The figure shows three views and two pictorial views of one solid part (mm, origin at its lowest corner). Answer the questions. A direction names the side the tool comes from. Round coordinates to 2 decimals unless told otherwise and drop trailing zeros. Write each loop counter-clockwise with the first axis right and the second up, starting at its lowest first coordinate (ties: lowest second). Pieces come first, ordered by that corner, then holes.
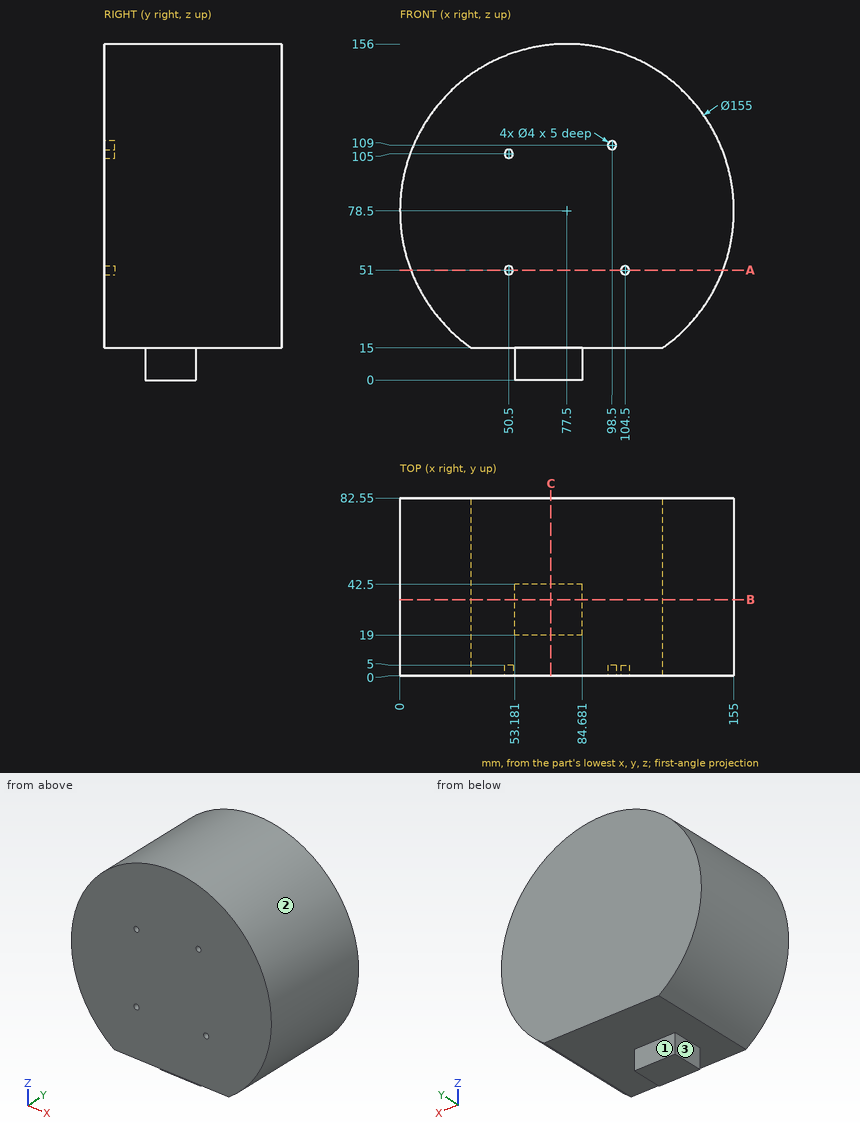
Q1. Section A-A (z = 51) is taken. Determine the outline of the cut face in (x, y).
Verdict:
outline: (5.04, 0) - (48.5, 0) - (48.5, 5) - (52.5, 5) - (52.5, 0) - (102.5, 0) - (102.5, 5) - (106.5, 5) - (106.5, 0) - (149.96, 0) - (149.96, 82.55) - (5.04, 82.55) - close
Q2. Section C-C (x = 70) is taken. Determine the outline of the cut face in (y, z).
Verdict:
outline: (0, 15) - (19, 15) - (19, 0) - (42.5, 0) - (42.5, 15) - (82.55, 15) - (82.55, 155.64) - (0, 155.64) - close
Q3. Section B-B (y = 35.5) is taken. Determine the outline of the cut face in (x, z).
Verdict:
outline: (33.07, 15) - (53.18, 15) - (53.18, 0) - (84.68, 0) - (84.68, 15) - (121.93, 15) arc R77.5 ccw (long way) to start
Q4. Straight lines are drawn through the part: probe 1 along Z at (x, y) = (50.5, 3.1) (1 decimal); probe 2 along Z at (x, y) = (77, 53); probe 3 along X at (y, z) = (2, 105). For each, find the intervals that lie inside material, in ascending order.
Verdict:
probe 1: z = 15 to 49, 53 to 103, 107 to 151.1
probe 2: z = 15 to 156
probe 3: x = 4.67 to 48.5, 52.5 to 150.33
Q5. Flat-ended cylindrical pins translate along their axes: pin 1 Ø2 at (x, y) = (125, 70.5) entering from -Z; pin 2 Ø4 at (x, z) = (82.5, 58.5) entering from -Y; pin 3 Ø4 at (y, z) = (41.5, 133) entering from -X; pin 4 Ø7.5 at (y, z) = (33.5, 8) entering from -X. Find the tip coordinate at first contact, or state that the pin passes through.
Verdict:
pin 1: stops at z = 16.5
pin 2: stops at y = 0
pin 3: stops at x = 20.49
pin 4: stops at x = 53.18
Q6. Which of the six approach directions +Z, -Z, +X, -X, +Y, -Y give full straight-line access (tool end or side, diameter ignored) to the marked faces 1, 2 and 3?
Verdict:
face 1: -Z, +X, -X, +Y
face 2: +Y, -Y
face 3: -Z, -X, +Y, -Y
